For this review, take the finished solid that the model builds, in its own axes (mm). A direction names the side the tool comes from. Give positions to 0.01 mm unless a question says otherwise; leave off trailing zeros. Order: outer loops, then holes, each group sorted by start corner. A loop starts at its lowest first (then second) coordinate and runs counter-clockwise, first axis right, second up. Notation, with made-up numbers: (19.25, 28.5) - (38.25, 28.5) arc R24 ccw to (38.25, 46.5) - close; hole circle Ø4 at (76.5, -3). An arc over 180 degrees is marked (long way). Use a Markdown table: item, result. Add a question column.
1) Machinability: for faces 4 (the face through (5.215, -23.114, 2.958)), 5 (the face through (-20, 0, 33)), 6 (the face through (-21, 22.5, 2)), which of the approach directions +Z, -Z, +X, -X, +Y, -Y give a long, thin tool a straight path to every point of the face, cutting with its end or side? Answer none if there is none.
2) We need section A-A on z = 15.5. Write out the cut boundary in (x, y).
3) Clearance check with flat-ended pins moving along their axes: P1, Ø2, axis at x = -16, y = 20, coming from the -Z side; P2, Ø3, axis at x = -4, y = -9.5, coming from the +Z side; P3, Ø4.5, axis at x = 24, z = -0.5, coming from the -Y side. State where each tip first meets the part, or that it passes through.
4) We need section D-D on y = -24.75. Write out the cut boundary in (x, z).
5) Mouldability with a two-part tool opening along X and no side actions: class faces 1 (the face through (12, 28, 23)), 2 (the face through (-12, -28, 23)), 3 (the face through (-5, 25, 6)) as released by +X, released by -X, zero draft, split by the parting line, or undercut.
6) Wall thickness on L1, parallel to Y at x = -5, z = 1.55; L2, parallel to Y at x = -16, z = -3; L3, parallel to Y at x = -24.25, z = 1.75: over which ranges is each line inside the solid? List them lowest first.
7) We need section B-B on x = 19. Write out the cut boundary in (y, z).
8) We need section C-C on x = 0. Write out the cut boundary in (y, z) (3 decimals).
```python
from build123d import *

# Parameters (mm, degrees)
SKETCH_1_W          = 25
SKETCH_1_H          = 60
EXTRUDE_1_DEPTH     = 35
SKETCH_2_W          = 20
SKETCH_2_H          = 40.5
CUT_EXTRUDE_1_DEPTH = 31.5
SKETCH_5_W          = 40
SKETCH_5_H          = 60
EXTRUDE_4_DEPTH     = 5
SKETCH_6_R          = 1.65
CUT_EXTRUDE_2_DEPTH = 6
SKETCH_10_W         = 15
SKETCH_10_H         = 45
EXTRUDE_7_DEPTH     = 16.75
SKETCH_18_R         = 1.25
CUT_EXTRUDE_4_DEPTH = 5
CUT_EXTRUDE_START   = -4
SKETCH_17_R         = 1.65
CUT_EXTRUDE_3_DEPTH = 12
SKETCH_13_R         = 3.5
EXTRUDE_10_DEPTH    = 45
SKETCH_15_R         = 17
SKETCH_15_R_2       = 15
EXTRUDE_11_DEPTH    = 6
CHAMFER_START       = 30
CHAMFER_3_DEPTH     = 5
CHAMFER_START_2     = -1
CHAMFER_3_2_DEPTH   = 31


with BuildPart() as part:
    # 草圖1 → 填料-伸長1 (new body)
    with BuildSketch(Plane.XY):
        Rectangle(SKETCH_1_W, SKETCH_1_H)
    extrude(amount=EXTRUDE_1_DEPTH)

    # 草圖2 → 除料-伸長1 (cut)
    with BuildSketch(Plane(origin=(0, 0, 0), x_dir=(-1, 0, 0), z_dir=(0, 0, -1))):
        Rectangle(SKETCH_2_W, SKETCH_2_H)
    extrude(amount=-CUT_EXTRUDE_1_DEPTH, mode=Mode.SUBTRACT)

    # 草圖5 → 填料-伸長4 (add)
    with BuildSketch(Plane.XY.offset(35)):
        Rectangle(SKETCH_5_W, SKETCH_5_H)
    extrude(amount=-EXTRUDE_4_DEPTH)

    # 草圖6 → 除料-伸長2 (cut)
    with BuildSketch(Plane(origin=(0, 0, 0), x_dir=(-1, 0, 0), z_dir=(0, 0, -1))):
        with Locations((5, 24.75)):
            Circle(SKETCH_6_R)
        with Locations((-5, 24.75)):
            Circle(SKETCH_6_R)
        with Locations((-5, -24.75)):
            Circle(SKETCH_6_R)
        with Locations((5, -24.75)):
            Circle(SKETCH_6_R)
    extrude(amount=-CUT_EXTRUDE_2_DEPTH, mode=Mode.SUBTRACT)

    # 草圖10 → 填料-伸長7 (add)
    with BuildSketch(Plane.ZY.offset(12.5)):
        with Locations((2.5, 0)):
            Rectangle(SKETCH_10_W, SKETCH_10_H)
    extrude_7 = extrude(amount=EXTRUDE_7_DEPTH)

    # 草圖18 → 除料-伸長4 (cut)
    with BuildSketch(Plane(origin=(0, 0, -5), x_dir=(-1, 0, 0), z_dir=(0, 0, -1))):
        with Locations((16, -20)):
            Circle(SKETCH_18_R)
        with Locations((16, 20)):
            Circle(SKETCH_18_R)
    cut_extrude_4 = extrude(amount=-CUT_EXTRUDE_4_DEPTH, mode=Mode.SUBTRACT)

    # 草圖17 → 除料-伸長3 (cut)
    with BuildSketch(Plane(origin=(0, 0, 0), x_dir=(-1, 0, 0), z_dir=(0, 0, -1)).offset(CUT_EXTRUDE_START)):
        with Locations(Location((24.25, 0, 0), (0, 0, 180))):
            Circle(SKETCH_17_R)
        with Locations(Location((24.25, -15, 0), (0, 0, 180))):
            Circle(SKETCH_17_R)
        with Locations(Location((24.25, 15, 0), (0, 0, 180))):
            Circle(SKETCH_17_R)
    cut_extrude_3 = extrude(amount=CUT_EXTRUDE_3_DEPTH, mode=Mode.SUBTRACT)

    # 鏡射1: 填料-伸長7, 除料-伸長4, 除料-伸長3 across plane
    add(extrude_7.mirror(Plane(origin=(0, 0, 0), x_dir=(0, 0, 1), z_dir=(1, 0, 0))))
    add(cut_extrude_4.mirror(Plane(origin=(0, 0, 0), x_dir=(0, 0, 1), z_dir=(1, 0, 0))), mode=Mode.SUBTRACT)
    add(cut_extrude_3.mirror(Plane(origin=(0, 0, 0), x_dir=(0, 0, 1), z_dir=(1, 0, 0))), mode=Mode.SUBTRACT)

    # 草圖13 → 填料-伸長10 (add)
    with BuildSketch(Plane.XY.offset(35)):
        with Locations(Location((0, 9.675, 0), (0, 0, 180))):
            Circle(SKETCH_13_R)
    extrude(amount=EXTRUDE_10_DEPTH)

    # 草圖15 → 填料-伸長11 (add)
    with BuildSketch(Plane.XY.offset(35)):
        with Locations(Location((0, 9.675, 0), (0, 0, 180))):
            Circle(SKETCH_15_R)
        with Locations((0, 9.675)):
            Circle(SKETCH_15_R_2, mode=Mode.SUBTRACT)
    extrude(amount=EXTRUDE_11_DEPTH)

    # 導角3: read off the stored shape, not the designer's step
    # 導角3 outline → 導角3 (cut)
    with BuildSketch(Plane.XY.offset(CHAMFER_START)):
        Polygon((20, 20), (20, 30), (10, 30), align=None)
        Polygon((20, -30), (20, -20), (10, -30), align=None)
        Polygon((-10, 30), (-20, 30), (-20, 20), align=None)
        Polygon((-10, -30), (-20, -20), (-20, -30), align=None)
    extrude(amount=CHAMFER_3_DEPTH, mode=Mode.SUBTRACT)

    # Chamfer 3 2 outline → Chamfer 3 2 (cut)
    with BuildSketch(Plane.XY.offset(CHAMFER_START_2)):
        Polygon((10, 30), (12.5, 27.5), (12.5, 30), align=None)
        Polygon((12.5, -30), (12.5, -27.5), (10, -30), align=None)
        Polygon((-12.5, 27.5), (-10, 30), (-12.5, 30), align=None)
        Polygon((-12.5, -30), (-10, -30), (-12.5, -27.5), align=None)
    extrude(amount=CHAMFER_3_2_DEPTH, mode=Mode.SUBTRACT)


solid = part.part
```
Checked values:
| question | item | result |
|---|---|---|
| 1 | face 4 | -Z |
| 1 | face 5 | +Z, -X, +Y, -Y |
| 1 | face 6 | -Z, -X, +Y |
| 2 | outline | (-12.5, -27.5) - (-10, -30) - (10, -30) - (12.5, -27.5) - (12.5, 27.5) - (10, 30) - (-10, 30) - (-12.5, 27.5) - close; hole (-10, -20.25) - (10, -20.25) - (10, 20.25) - (-10, 20.25) - close |
| 3 | P1 | z = 0 |
| 3 | P2 | z = 35 |
| 3 | P3 | y = -22.5 |
| 4 | outline | (-15.25, 30) - (-12.5, 30) - (-12.5, 0) - (-6.65, 0) - (-6.65, 6) - (-3.35, 6) - (-3.35, 0) - (3.35, 0) - (3.35, 6) - (6.65, 6) - (6.65, 0) - (12.5, 0) - (12.5, 30) - (15.25, 30) - (15.25, 35) - (-15.25, 35) - close |
| 5 | face 1 | released by +X |
| 5 | face 2 | released by -X |
| 5 | face 3 | undercut |
| 6 | L1 | -30 to -26.4, -23.1 to -20.25, 20.25 to 23.1, 26.4 to 30 |
| 6 | L2 | -22.5 to -21.25, -18.75 to 18.75, 21.25 to 22.5 |
| 6 | L3 | -22.5 to -16.65, -13.35 to -1.65, 1.65 to 13.35, 16.65 to 22.5 |
| 7 | outline | (-22.5, -5) - (22.5, -5) - (22.5, 10) - (-22.5, 10) - close; (-21, 30) - (21, 30) - (21, 35) - (-21, 35) - close |
| 8 | outline | (-30, 0) - (-20.25, 0) - (-20.25, 30) - (20.25, 30) - (20.25, 0) - (30, 0) - (30, 35) - (26.675, 35) - (26.675, 41) - (24.675, 41) - (24.675, 35) - (13.175, 35) - (13.175, 80) - (6.175, 80) - (6.175, 35) - (-5.325, 35) - (-5.325, 41) - (-7.325, 41) - (-7.325, 35) - (-30, 35) - close |
